Can you work these out from the model? Positions are in its coordinate system, mm. Face numbers are marked on the shaded views. Round coordinates to 2 decimals unless told otherwise and drop trailing zeros. Write each loop counter-clockwise with the first axis right and the second up, starting at its lowest first coordinate (ties: lowest second). Pieces come first, ordered by that corner, then holes.
Q1. If we section it at C-C (z = -17): Please give me the cut outline in (x, y).
Q2. If we section it at A-A (z = 7): Please give me the cut outline in (x, y), plus the area to 3 significant figures.
Q3. I'm going to push flat-ended pins straight in: pin 1 Ø12 at (x, z) = (14.5, 0) entering from +Y; pin 2 Ø6 at (x, y) = (23.5, -16) entering from -Z; pin 3 Ø5 at (y, z) = (-13, -7) entering from +X; pin 4 Ø12 at (y, z) = (-16, 27) entering from -X. Where does each tip first touch, or does it pass through?
Q4. If we section it at B-B (x = -19.5): Please give me the cut outline in (y, z), plus the area to 3 significant figures.
Q5. We'd pull the mould along X, two halves only. Please class the marked faces 1, 2 and 3: +X half, -X half, draft (parallel to the pull), parting line (faces both ways), or undercut.
Q6. Please list where these lines run through material, in increasing order: line 1 along Z through (x, y) = (1, -8.5); line 2 along X through (y, z) = (-3.25, 8.5); line 3 along Z through (x, y) = (0.5, -18).
from build123d import *

# Parameters (mm, degrees)
F1_DEPTH = 25
F0_R     = 9.7528106777
F2_DEPTH = 25
F3_COUNT = 12


with BuildPart() as f1:
    # F0 (on Front) → F1 (new body)
    with BuildSketch(Plane.XZ):
        with BuildLine():
            ThreePointArc((35.2883561629, 1.0330273155), (27.4544642418, 24.8582881027), (7.0100539825, 39.385469638))
            ThreePointArc((7.0100539825, 39.385469638), (1.4007375004, 40.6889829464), (-4.3373688538, 41.1765419779))
            ThreePointArc((-4.3373688538, 41.1765419779), (-6.7990788962, 41.1329986982), (-9.2534905381, 40.9386386143))
            ThreePointArc((-9.2534905381, 40.9386386143), (-31.6478100439, -28.8686194646), (35.2883561629, 1.0330273155))
        make_face()
        with BuildLine():
            ThreePointArc((-4.85854148, 30.3700273155), (14.134700216, 22.5027690116), (22.00195852, 3.5095273155))
            ThreePointArc((22.00195852, 3.5095273155), (-22.4423355568, -16.7955618523), (-8.697145824, 30.0943270504))
            ThreePointArc((-8.697145824, 30.0943270504), (-6.7827876925, 30.3010135894), (-4.85854148, 30.3700273155))
        make_face(mode=Mode.SUBTRACT)
        with BuildLine():
            ThreePointArc((-9.2534905381, 40.9386386143), (-6.7990788962, 41.1329986982), (-4.3373688538, 41.1765419779))
            Line((-4.3373688538, 41.1765419779), (-5.4201926105, 45.7159504294))
            Line((-5.4201926105, 45.7159504294), (-7.7872149896, 45.7159504294))
            Line((-7.7872149896, 45.7159504294), (-9.2534905381, 40.9386386143))
        make_face()
    extrude(amount=F1_DEPTH)

    # F0 (on Front) → F2 (join)
    with BuildSketch(Plane.XZ):
        with BuildLine():
            ThreePointArc((-8.697145824, 30.0943270504), (-22.4423355568, -16.7955618523), (22.00195852, 3.5095273155))
            ThreePointArc((22.00195852, 3.5095273155), (14.134700216, 22.5027690116), (-4.85854148, 30.3700273155))
            ThreePointArc((-4.85854148, 30.3700273155), (-6.7827876925, 30.3010135894), (-8.697145824, 30.0943270504))
        make_face()
        with Locations((-4.85854148, 1.0330273155)):
            Circle(F0_R, mode=Mode.SUBTRACT)
    extrude(amount=F2_DEPTH)

    # F3: F1 ×12 about axis
    f3_axis = Axis((-4.85854148, 0, 1.0330273155), (0, -1, 0))


with BuildPart() as f1_1:
    add(f1.part)
    for i in range(1, F3_COUNT):
        add(f1.part.rotate(f3_axis, i * 360 / F3_COUNT))


solid = f1_1.part
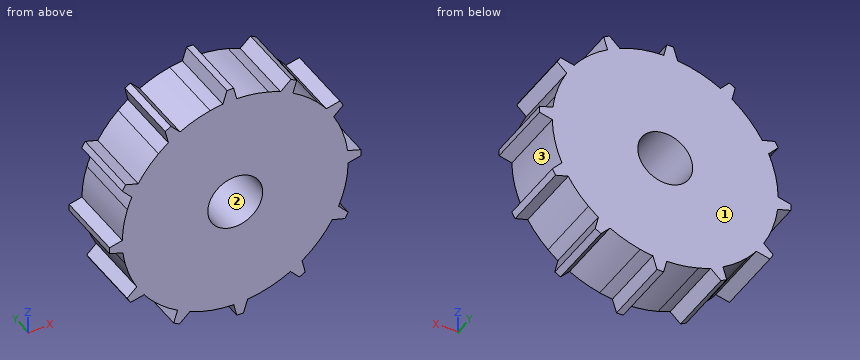
A:
1. outline: (-40.73, -25) - (33.65, -25) - (33.65, 0) - (-40.73, 0) - close
2. outline: (-44.56, -25) - (-12.57, -25) - (-12.57, 0) - (-44.56, 0) - close; (2.86, -25) - (34.84, -25) - (34.84, 0) - (2.86, 0) - close
2. area: 1,600 mm2
3. pin 1: stops at y = 0
3. pin 2: stops at z = -30.09
3. pin 3: stops at x = 34.91
3. pin 4: stops at x = -44.93
4. outline: (-25, -36.35) - (0, -36.35) - (0, 38.41) - (-25, 38.41) - close
4. area: 1,870 mm2
5. face 1: draft
5. face 2: undercut
5. face 3: +X half
6. line 1: z = -38.68 to -6.76, 8.83 to 40.75
6. line 2: x = -44.3 to -11.13, 1.42 to 34.59
6. line 3: z = -38.75 to -7.12, 9.18 to 40.82
